from build123d import *

# Parameters (mm, degrees)
SKETCH2_R           = 36.5
SKETCH2_R_2         = 2.5
BOSS_EXTRUDE1_DEPTH = 2
CHAMFER1_SIZE       = 2
FILLET1_R           = 0.5


with BuildPart() as part:
    # Sketch2 → Boss-Extrude1 (new body)
    with BuildSketch(Plane(origin=(0, 0, 0), x_dir=(1, 0, 0), z_dir=(0, 1, 0))):
        with Locations(Location((0, 0, 0), (0, 0, 270))):
            Circle(SKETCH2_R)
        with Locations(Location((0, 25.52, 0), (0, 0, 270))):
            Circle(SKETCH2_R_2, mode=Mode.SUBTRACT)
        with Locations(Location((24.270962296, 7.886113696, 0), (0, 0, 270))):
            Circle(SKETCH2_R_2, mode=Mode.SUBTRACT)
        with Locations(Location((15.000279639, -20.646113696, 0), (0, 0, 270))):
            Circle(SKETCH2_R_2, mode=Mode.SUBTRACT)
        with Locations(Location((-15.000279639, -20.646113696, 0), (0, 0, 270))):
            Circle(SKETCH2_R_2, mode=Mode.SUBTRACT)
        with Locations(Location((-24.270962296, 7.886113696, 0), (0, 0, 270))):
            Circle(SKETCH2_R_2, mode=Mode.SUBTRACT)
    extrude(amount=BOSS_EXTRUDE1_DEPTH)

    # Chamfer1
    chamfer1_edges = [part.edges().sort_by_distance(p)[0] for p in [
        (-24.270962296, 2, -10.386113696),
        (-15.000279639, 2, 18.146113696),
        (15.000279639, 2, 18.146113696),
        (24.270962296, 2, -10.386113696),
        (0, 2, -28.02),
    ]]
    chamfer(chamfer1_edges, length=CHAMFER1_SIZE - 0.0001)  # a hair under: the kernel refuses the full size

    # Fillet1
    fillet1_edges = [part.edges().sort_by_distance(p)[0] for p in [
        (0, 2, -36.5),
    ]]
    fillet(fillet1_edges, radius=FILLET1_R)


solid = part.part
For this review, take the finished solid that the model builds, in its own axes (mm). Give positions to 0.01 mm unless a question says otherwise; leave off trailing zeros. Loops run counter-clockwise (first coordinate to the right, second up) from the corner with the lowest first, then second, coordinate; pieces in that order, holes last. Notation, with made-up numbers: (-31.5, 67.5) - (15.5, 67.5) arc R13 ccw to (15.5, 85.5) - close; hole circle Ø11 at (30.25, 34). An arc over 180 degrees is marked (long way). Write each question's results on one line, items separated by ' | '.
(1) Take a section at B-B (y = 0.8). Give the boundary of the cut face in (x, z).
Conclusion:
outline: circle Ø73 at (0, 0); hole circle Ø6.6 at (-24.27, -7.89); hole circle Ø6.6 at (-15, 20.65); hole circle Ø6.6 at (0, -25.52); hole circle Ø6.6 at (15, 20.65); hole circle Ø6.6 at (24.27, -7.89)
(2) For line 1 along X through (y, z) = (0.55, -7); line 2 along Z through (x, y) = (-16.5, 0.45); line 3 along Z through (x, y) = (14, 0.1), list the stretches that pass through material, from the lowest coordinate up.
Conclusion:
line 1: -35.82 to -27.19, -21.35 to 21.35, 27.19 to 35.82 | line 2: -32.56 to 18.11, 23.19 to 32.56 | line 3: -33.71 to 18.25, 23.05 to 33.71
(3) For pin 1 Ø4.5 at (x, z) = (24.27, -7.89) entering from +Y; pin 2 Ø8 at (x, z) = (15, 20.65) entering from +Y, all flat-tipped, find the tip position at first contact; note any pin that passes through.
Conclusion:
pin 1: through | pin 2: y = 1.5
